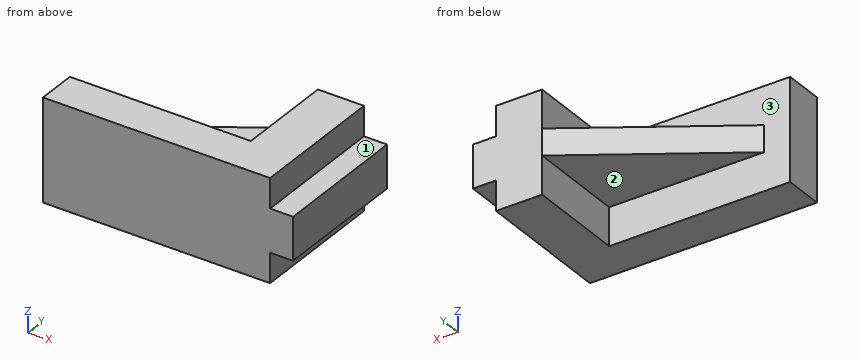
from build123d import *

# Parameters (mm, degrees)
SKETCH1_W               = 76
SKETCH1_H               = 42
BOSS_EXTRUDE1_DEPTH     = 15.5
SKETCH2_W               = 9
SKETCH2_H               = 42
CUT_EXTRUDE1_DEPTH      = 7
CUT_EXTRUDE2_DEPTH      = 93.200867675
CUT_EXTRUDE2_DEPTH_BACK = 93.200867675
SKETCH3_W               = 55
SKETCH3_H               = 30
BOSS_EXTRUDE2_DEPTH     = 4


with BuildPart() as part:
    # Sketch1 → Boss-Extrude1 (new, symmetric)
    with BuildSketch(Plane.XY):
        with Locations((38, 21)):
            Rectangle(SKETCH1_W, SKETCH1_H)
    extrude(amount=BOSS_EXTRUDE1_DEPTH, both=True)

    # Sketch2 → Cut-Extrude1 (cut)
    with BuildSketch(Plane(origin=(76, 0, 0), x_dir=(0, 0, -1), z_dir=(1, 0, 0))):
        with Locations((-11, 21)):
            Rectangle(SKETCH2_W, SKETCH2_H)
        with Locations((11, 21)):
            Rectangle(SKETCH2_W, SKETCH2_H)
    extrude(amount=-CUT_EXTRUDE1_DEPTH, mode=Mode.SUBTRACT)

    # Sketch3 → Cut-Extrude2 (cut, two sides: drawn at the far end of the back side and taken through both)
    with BuildSketch(Plane.XY.offset(15.5).offset(-CUT_EXTRUDE2_DEPTH_BACK)):
        with Locations((27.5, 27)):
            Rectangle(SKETCH3_W, SKETCH3_H)
    extrude(amount=CUT_EXTRUDE2_DEPTH + CUT_EXTRUDE2_DEPTH_BACK, mode=Mode.SUBTRACT)

    # Sketch5 → Boss-Extrude2 (add, symmetric)
    with BuildSketch(Plane.XY):
        Polygon((55, 42), (8, 12), (55, 12), (55, 12.687234068), align=None)
    extrude(amount=BOSS_EXTRUDE2_DEPTH, both=True)


solid = part.part
For this review, take the finished solid that the model builds, in its own axes (mm). Face numbers are marked on the shaded views. A direction names the side the tool comes from. Coordinates: 2 decimals unless noted, no trailing zeros. Loops run counter-clockwise (first coordinate to the right, second up) from the corner with the lowest first, then second, coordinate; pieces in that order, holes last. Notation, with made-up numbers: (46, 5.25) - (68, 5.25) arc R24 cw to (68, 23.25) - close; hole circle Ø10 at (1, -2). An arc over 180 degrees is marked (long way). Return JSON: item names as keys, results as strings.
Item 1: Take a section at B-B (z = 1.5). Give the boundary of the cut face in (x, y).
Determined:
{"outline": "(0, 0) - (76, 0) - (76, 42) - (55, 42) - (8, 12) - (0, 12) - close"}
Item 2: For line 1 (X direction, y = 20, z = -10); line 2 (X direction, y = 9, z = 10); line 3 (Z direction, x = 28.5, y = 24), list the stretches that pass through material, from the lowest coordinate up.
Determined:
{"line 1": "x = 55 to 69", "line 2": "x = 0 to 69", "line 3": "z = -4 to 4"}
Item 3: Take a section at D-D (y = 28.5). Give the boundary of the cut face in (x, z).
Determined:
{"outline": "(33.85, -4) - (55, -4) - (55, -15.5) - (69, -15.5) - (69, -6.5) - (76, -6.5) - (76, 6.5) - (69, 6.5) - (69, 15.5) - (55, 15.5) - (55, 4) - (33.85, 4) - close"}
Item 4: For the marked faces 1, 2 and 3, list the 3-axis set-ups (+Z, -Z, +X, -X, +Y, -Y) from which the entire face can be reached by the end or side of a thin tool; tool diameter is ignored.
Determined:
{"face 1": "+Z, +X, +Y, -Y", "face 2": "-Z, -X, +Y", "face 3": "-X, +Y"}
Item 5: Take a section at C-C (x = 51). Give the boundary of the cut face in (y, z), then the cut area to 3 significant figures.
Determined:
{"outline": "(0, -15.5) - (12, -15.5) - (12, -4) - (39.45, -4) - (39.45, 4) - (12, 4) - (12, 15.5) - (0, 15.5) - close", "area": "592 mm2"}
Item 6: Take a section at A-A (y = 33). Give the boundary of the cut face in (x, z).
Determined:
{"outline": "(40.9, -4) - (55, -4) - (55, -15.5) - (69, -15.5) - (69, -6.5) - (76, -6.5) - (76, 6.5) - (69, 6.5) - (69, 15.5) - (55, 15.5) - (55, 4) - (40.9, 4) - close"}
Item 7: Insertion check: pin 1 (15.5 mm diameter, centred on x = 39.5, z = 1, fed in from +Y); pin 2 (24 mm diameter, centred on x = 20, y = 32.5, fed in from -Z); pin 3 (12 mm diameter, centred on x = 52, z = 2, fed in from +Y); pin 4 (7.5 mm diameter, centred on x = 73.5, y = 12, fed in from -Z). Each pin has a flat end and moves straight along its axis. Give the tip position at first contact, or say it passes through.
Determined:
{"pin 1": "stops at y = 37.05", "pin 2": "stops at z = -4", "pin 3": "stops at y = 42", "pin 4": "stops at z = -6.5"}
